Job drawing, mm, ordinate dimensions from the low corner. One solid piece. A direction names the side the tool comes from. Give positions to 0.01 mm unless a question says otherwise; leave off trailing zeros. Write each loop counter-clockwise with the first axis right and the second up, starting at its lowest first coordinate (ties: lowest second). Pieces come first, ordered by that corner, then holes. Notation, with made-up numbers: (38.5, -23) - (88.5, -23) arc R25 ccw to (88.5, 9) - close; hole circle Ø5 at (-20.75, 1.5). An arc over 180 degrees is marked (long way). Use a Markdown table: item, result. Add a question column.
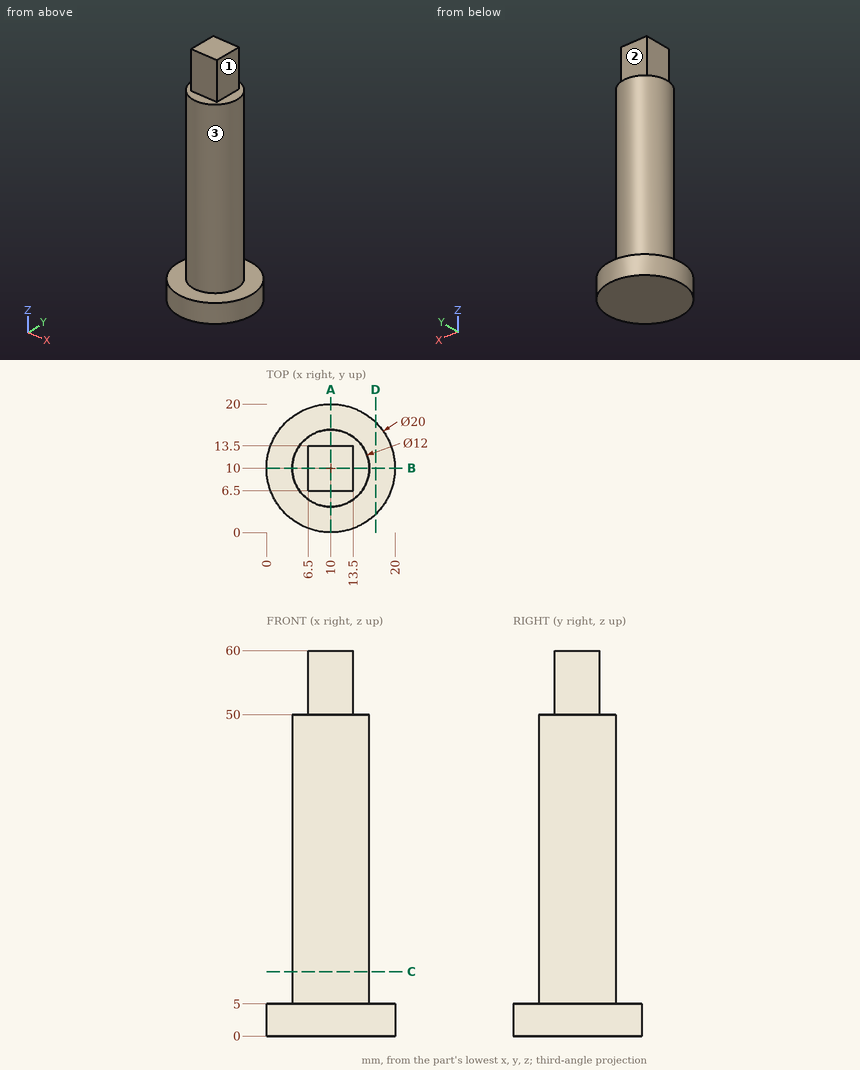
(1) Probe probe 1 along Z at (x, y) = (6.25, 10.5); probe 2 along Z at (x, y) = (3.75, 14); probe 3 along X at (y, z) = (12, 35). List the from-to ranges inside material, lowest first. Write a range as [from, to].
(2) Which spindle directions (+Z, -Z, +X, -X, +Y, -Y) get a long thin tool onto all of the face, cutting with end or side? Do the marked faces 1, 2 and 3. Say none if no direction does.
(3) Band-saw the part on D-D (x = 17). Write the cut outline in (y, z), then the cut area to 3 significant figures.
(4) Flat gauge pins, fed straight in: pin 1 (1.5 mm diameter, centred on y = 16, z = 52.5, fed in from +X); pin 2 (12 mm diameter, centred on x = 17.5, z = 51, fed in from -Y); pin 3 (3.5 mm diameter, centred on x = 9.5, z = 54, fed in from -Y); pin 4 (5 mm diameter, centred on y = 17.5, z = 26.5, fed in from -X). Where does each tip first touch, or does it go through?
(5) Band-saw the part on C-C (z = 10). Write the cut outline in (x, y), then the cut area to 3 significant figures.
(6) Band-saw the part on A-A (x = 10). Write the cut outline in (y, z).
Model answer:
| question | item | result |
|---|---|---|
| 1 | probe 1 | z = [0, 50] |
| 1 | probe 2 | z = [0, 5] |
| 1 | probe 3 | x = [4.34, 15.66] |
| 2 | face 1 | +Z, +X, +Y, -Y |
| 2 | face 2 | +Z, +X, -X, +Y |
| 2 | face 3 | +Z |
| 3 | outline | (2.86, 0) - (17.14, 0) - (17.14, 5) - (2.86, 5) - close |
| 3 | area | 71.4 mm^2 |
| 4 | pin 1 | passes through |
| 4 | pin 2 | stops at y = 4.21 |
| 4 | pin 3 | stops at y = 6.5 |
| 4 | pin 4 | stops at x = 6.68 |
| 5 | outline | circle Ø12 at (10, 10) |
| 5 | area | 113 mm^2 |
| 6 | outline | (0, 0) - (20, 0) - (20, 5) - (16, 5) - (16, 50) - (13.5, 50) - (13.5, 60) - (6.5, 60) - (6.5, 50) - (4, 50) - (4, 5) - (0, 5) - close |
